Verification items for the finished model (mm, model axes). A direction names the side the tool comes from. Give positions to 0.01 mm unless a question says otherwise; leave off trailing zeros. Loops run counter-clockwise (first coordinate to the right, second up) from the corner with the lowest first, then second, coordinate; pieces in that order, holes last. Notation, with made-up numbers: M -24,48 L 11,48 A35 cw 11,83 Z; hole C 22.5,63.25 d7. An arc over 180 degrees is marked long. Use CSV: the item, a comma, the result in double quotes.
from build123d import *

# Parameters (mm, degrees)
ESQUISSE2_W          = 7.2
ESQUISSE2_H          = 2.5
BOITIER_DEPTH        = 4.1
FENETRECAPTEUR_START = -1.45
ESQUISSE4_R          = 0.8
FENETRECAPTEUR_DEPTH = 0.1
PATTES_DEPTH         = 0.15
PLIAGE_START         = -5
PLIAGE_1_OUTLINE_W   = 7.2
PLIAGE_1_OUTLINE_H   = 4.1
PLIAGE_1_DEPTH       = 4.301040764
PLIAGE_START_2       = -0.698959236
PLIAGE_1_2_OUTLINE_R = 0.8
PLIAGE_1_2_DEPTH     = 0.1
PLIAGE_START_3       = -0.598959236
PLIAGE_1_3_OUTLINE_W = 7.2
PLIAGE_1_3_OUTLINE_H = 4.1
PLIAGE_1_3_DEPTH     = 2.4
PLIAGE_1_4_OUTLINE_W = 7.2
PLIAGE_1_4_OUTLINE_H = 4.1
PLIAGE_1_4_OUTLINE_R = 0.8
PLIAGE_1_4_DEPTH     = 0.1
PLIAGE_START_4       = -3.6
PLIAGE_1_5_DEPTH     = 7.2
PLIAGE_START_5       = -2.813242849
PLIAGE_1_6_DEPTH     = 0.546485698
PLIAGE_START_6       = -1.543242849
PLIAGE_1_7_DEPTH     = 0.546485698
PLIAGE_START_7       = 0.996757151
PLIAGE_1_8_DEPTH     = 0.546485698
PLIAGE_START_8       = 2.266757151
PLIAGE_1_9_DEPTH     = 0.546485698
PLIAGE_START_9       = 0.601040763
PLIAGE_1_10_DEPTH    = 0.300000001


with BuildPart() as part:
    # Esquisse2 → Boitier (new body)
    with BuildSketch(Plane.XY):
        with Locations((0, -0.2)):
            Rectangle(ESQUISSE2_W, ESQUISSE2_H)
    extrude(amount=BOITIER_DEPTH)

    # Esquisse4 → FenetreCapteur (cut)
    with BuildSketch(Plane(origin=(0, 0, 0), x_dir=(1, 0, 0), z_dir=(0, 1, 0)).offset(FENETRECAPTEUR_START)):
        with Locations(Location((-1.27, -2.3, 0), (0, 0, 180))):
            Circle(ESQUISSE4_R)
        with Locations(Location((1.27, -2.3, 0), (0, 0, 180))):
            Circle(ESQUISSE4_R)
    extrude(amount=FENETRECAPTEUR_DEPTH, mode=Mode.SUBTRACT)

    # Esquisse5 → Pattes (add, symmetric)
    with BuildSketch(Plane(origin=(0, 0, 0), x_dir=(1, 0, 0), z_dir=(0, 1, 0))):
        Polygon((2.79, 2.2), (2.79, 2.9), (2.29, 2.9), (2.29, 2.2), (2.053248267, 2.2), (2.053248267, 1.724539267), (2.266757151, 1.724539267), (2.266757151, 0.7), (2.002499851, 0), (2.991852509, 0), (2.813242849, 0.7), (2.813242849, 1.724539267), (3.170462168, 1.724539267), (3.170462168, 2.2), align=None)
        Polygon((1.52, 2.2), (1.52, 2.9), (1.02, 2.9), (1.02, 2.2), (0.639537832, 2.2), (0.639537832, 1.724539267), (0.996757151, 1.724539267), (0.996757151, 0.7), (0.818147491, 0), (1.807500149, 0), (1.543242849, 0.7), (1.543242849, 1.724539267), (1.756751733, 1.724539267), (1.756751733, 2.2), align=None)
        Polygon((-1.02, 2.2), (-1.02, 2.9), (-1.52, 2.9), (-1.52, 2.2), (-1.756751733, 2.2), (-1.756751733, 1.724539267), (-1.543242849, 1.724539267), (-1.543242849, 0.7), (-1.807500149, 0), (-0.818147491, 0), (-0.996757151, 0.7), (-0.996757151, 1.724539267), (-0.639537832, 1.724539267), (-0.639537832, 2.2), align=None)
        Polygon((-2.29, 2.2), (-2.29, 2.9), (-2.79, 2.9), (-2.79, 2.2), (-3.170462168, 2.2), (-3.170462168, 1.724539267), (-2.813242849, 1.724539267), (-2.813242849, 0.7), (-2.991852509, 0), (-2.002499851, 0), (-2.266757151, 0.7), (-2.266757151, 1.724539267), (-2.053248267, 1.724539267), (-2.053248267, 2.2), align=None)
    extrude(amount=PATTES_DEPTH, both=True)

    # Pliage 1: read off the stored shape, not the designer's step
    # Pliage 1 outline → Pliage 1 (cut)
    with BuildSketch(Plane(origin=(0, 0, 0), x_dir=(1, 0, 0), z_dir=(0, 0.707106781186546, -0.707106781186549)).offset(PLIAGE_START)):
        with Locations((0, -2.236827202)):
            Rectangle(PLIAGE_1_OUTLINE_W, PLIAGE_1_OUTLINE_H)
    extrude(amount=PLIAGE_1_DEPTH, mode=Mode.SUBTRACT)

    # Pliage 1 2 outline → Pliage 1 2 (cut)
    with BuildSketch(Plane(origin=(0, 0, 0), x_dir=(1, 0, 0), z_dir=(0, 0.707106781186546, -0.707106781186549)).offset(PLIAGE_START_2)):
        with Locations((-1.27, -2.486827202)):
            Circle(PLIAGE_1_2_OUTLINE_R)
        with Locations((1.27, -2.486827202)):
            Circle(PLIAGE_1_2_OUTLINE_R)
    extrude(amount=PLIAGE_1_2_DEPTH, mode=Mode.SUBTRACT)

    # Pliage 1 3 outline → Pliage 1 3 (add)
    with BuildSketch(Plane(origin=(0, 0, 0), x_dir=(1, 0, 0), z_dir=(0, 0.707106781186546, -0.707106781186549)).offset(PLIAGE_START_3)):
        with Locations((0, -2.236827202)):
            Rectangle(PLIAGE_1_3_OUTLINE_W, PLIAGE_1_3_OUTLINE_H)
    extrude(amount=PLIAGE_1_3_DEPTH)

    # Pliage 1 4 outline → Pliage 1 4 (add)
    with BuildSketch(Plane(origin=(0, 0, 0), x_dir=(1, 0, 0), z_dir=(0, 0.707106781186546, -0.707106781186549)).offset(PLIAGE_START_2)):
        with Locations((0, -2.236827202)):
            Rectangle(PLIAGE_1_4_OUTLINE_W, PLIAGE_1_4_OUTLINE_H)
        with Locations((-1.27, -2.486827202)):
            Circle(PLIAGE_1_4_OUTLINE_R, mode=Mode.SUBTRACT)
        with Locations((1.27, -2.486827202)):
            Circle(PLIAGE_1_4_OUTLINE_R, mode=Mode.SUBTRACT)
    extrude(amount=PLIAGE_1_4_DEPTH)

    # Pliage 1 5 outline → Pliage 1 5 (cut)
    with BuildSketch(Plane.YZ.offset(PLIAGE_START_4)):
        with BuildLine():
            Line((0.021781873, -0.828218127), (0.15, -0.7))
            Line((0.15, -0.7), (0.15, 0))
            Line((0.15, 0), (0.264213563, 0))
            Line((0.264213563, 0), (-1.35, 1.614213563))
            Line((-1.35, 1.614213563), (-1.45, 1.714213563))
            Line((-1.45, 1.714213563), (-1.45, 0))
            Line((-1.45, 0), (-0.15, 0))
            Line((-0.15, 0), (-0.15, -1.242936254))
            ThreePointArc((-0.15, -1.242936254), (-0.105355346, -1.018492421), (0.021781873, -0.828218127))
        make_face()
    extrude(amount=PLIAGE_1_5_DEPTH, mode=Mode.SUBTRACT)

    # Pliage 1 6 outline → Pliage 1 6 (add)
    with BuildSketch(Plane.YZ.offset(PLIAGE_START_5)):
        with BuildLine():
            Line((0.769238816, -0.505025253), (0.557106781, -0.292893218))
            Line((0.557106781, -0.292893218), (0.15, -0.7))
            Line((0.15, -0.7), (0.15, -1.242936254))
            ThreePointArc((0.15, -1.242936254), (0.171808514, -1.133297451), (0.233913907, -1.040350162))
            Line((0.233913907, -1.040350162), (0.769238816, -0.505025253))
        make_face()
    extrude(amount=PLIAGE_1_6_DEPTH)

    # Pliage 1 7 outline → Pliage 1 7 (add)
    with BuildSketch(Plane.YZ.offset(PLIAGE_START_6)):
        with BuildLine():
            Line((0.769238816, -0.505025253), (0.557106781, -0.292893218))
            Line((0.557106781, -0.292893218), (0.15, -0.7))
            Line((0.15, -0.7), (0.15, -1.242936254))
            ThreePointArc((0.15, -1.242936254), (0.171808514, -1.133297451), (0.233913907, -1.040350162))
            Line((0.233913907, -1.040350162), (0.769238816, -0.505025253))
        make_face()
    extrude(amount=PLIAGE_1_7_DEPTH)

    # Pliage 1 8 outline → Pliage 1 8 (add)
    with BuildSketch(Plane.YZ.offset(PLIAGE_START_7)):
        with BuildLine():
            Line((0.769238816, -0.505025253), (0.557106781, -0.292893218))
            Line((0.557106781, -0.292893218), (0.15, -0.7))
            Line((0.15, -0.7), (0.15, -1.242936254))
            ThreePointArc((0.15, -1.242936254), (0.171808514, -1.133297451), (0.233913907, -1.040350162))
            Line((0.233913907, -1.040350162), (0.769238816, -0.505025253))
        make_face()
    extrude(amount=PLIAGE_1_8_DEPTH)

    # Pliage 1 9 outline → Pliage 1 9 (add)
    with BuildSketch(Plane.YZ.offset(PLIAGE_START_8)):
        with BuildLine():
            Line((0.769238816, -0.505025253), (0.557106781, -0.292893218))
            Line((0.557106781, -0.292893218), (0.15, -0.7))
            Line((0.15, -0.7), (0.15, -1.242936254))
            ThreePointArc((0.15, -1.242936254), (0.171808514, -1.133297451), (0.233913907, -1.040350162))
            Line((0.233913907, -1.040350162), (0.769238816, -0.505025253))
        make_face()
    extrude(amount=PLIAGE_1_9_DEPTH)

    # Pliage 1 10 outline → Pliage 1 10 (add)
    with BuildSketch(Plane(origin=(0, 0, 0), x_dir=(1, 0, 0), z_dir=(0, 0.707106781186546, -0.707106781186549)).offset(PLIAGE_START_9)):
        Polygon((2.813242849, 0.513172798), (2.813242849, -0.186827202), (2.991852509, -0.186827202), align=None)
        Polygon((-2.991852509, -0.186827202), (-2.813242849, -0.186827202), (-2.813242849, 0.513172798), align=None)
        Polygon((-2.266757151, -0.186827202), (-2.002499851, -0.186827202), (-2.266757151, 0.513172798), align=None)
        Polygon((-1.807500149, -0.186827202), (-1.543242849, -0.186827202), (-1.543242849, 0.513172798), align=None)
        Polygon((-0.996757151, -0.186827202), (-0.818147491, -0.186827202), (-0.996757151, 0.513172798), align=None)
        Polygon((0.818147491, -0.186827202), (0.996757151, -0.186827202), (0.996757151, 0.513172798), align=None)
        Polygon((1.543242849, -0.186827202), (1.807500149, -0.186827202), (1.543242849, 0.513172798), align=None)
        Polygon((2.266757151, 0.513172798), (2.002499851, -0.186827202), (2.266757151, -0.186827202), align=None)
    extrude(amount=PLIAGE_1_10_DEPTH)


solid = part.part
(1) Scan lines: L1, parallel to X at y = 0.1, z = -2; L2, parallel to Z at x = 2.25, y = 2.25; L3, parallel to Y at x = 1.5, z = 0.5. Record each from-to range of solid material in increasing order. Write a range as from..to.
Calculated:
L1,"x = -3.17..-2.05, -1.76..-0.64, 0.64..1.76, 2.05..3.17"
L2,"z = -0.3..3.24"
L3,"y = -0.24..3.05"
(2) Tool access check on faces 1 (the flat face through (3, -0.15, -2)), 2 (the flat face through (-1, 0.15, -2)), 3 (the flat face through (-0.05, 1.07, 2.06)). Record the directions out of +Z, -Z, +X, -X, +Y, -Y that give a thin tool (end or side, any length) a straight path to the whole face; none if there is none.
Calculated:
face 1,"-Z, +X, -X, -Y"
face 2,"-Z, +X, -X, +Y"
face 3,"+Z, +X, -X, -Y"
(3) Section check B-B on y = 3.35. Record the cut outline in (x, z).
Calculated:
outline,"M -3.6,0.8 L 3.6,0.8 L 3.6,2.71 L -3.6,2.71 Z"
(4) Depth check by flat-ended pin: pin 1 Ø1.2 at (x, z) = (1.5, -2) entering from -Y; pin 2 Ø1 at (x, y) = (-1.5, 4) entering from +Z. Enter the tip coordinate at first touch or a pass-through.
Calculated:
pin 1,"stops at y = -0.15"
pin 2,"stops at z = 2.56"
(5) Mould release check, pull along X, two halves, no side actions. Record for faces 4 (the flat face through (1.259, 1.327, 2.174)), 5 (the flat face through (-3.6, 2, 1)), 6 (the flat face through (3, 0.15, -2)): released by +X, released by -X, zero draft, split by the parting line, or undercut.
Calculated:
face 4,"undercut"
face 5,"released by -X"
face 6,"zero draft"
(6) Section check C-C on z = 0.25. Record the cut outline in (x, y).
Calculated:
outline,"M -3.6,0.01 L 3.6,0.01 L 3.6,2.8 L -3.6,2.8 Z"
(7) Section check A-A on x = -2.5. Record the cut outline in (y, z).
Calculated:
outline,"M -0.36,0.63 L 0.56,-0.29 L 0.02,-0.83 A0.59 ccw -0.15,-1.24 L -0.15,-2.9 L 0.15,-2.9 L 0.15,-1.24 A0.29 cw 0.23,-1.04 L 0.77,-0.51 L 1.41,-1.14 L 4.3,1.76 L 2.54,3.53 Z"
